The listing builds one solid part. Answer for the finished solid, in the listing's coordinates (mm). Coordinates: 2 decimals unless noted, no trailing zeros. Write each loop counter-clockwise with the first axis right and the second up, starting at its lowest first coordinate (ties: lowest second). Pieces come first, ordered by that corner, then holes.
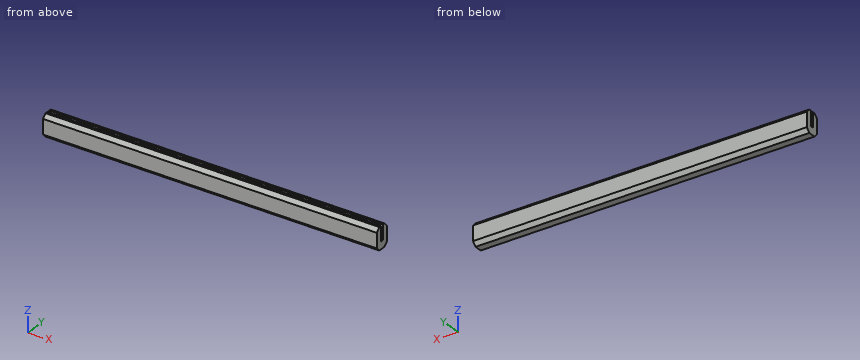
from build123d import *

# Parameters (mm, degrees)
F0_W     = 90
F0_H     = 1.625
F0_H_2   = 0.75
F1_DEPTH = 2
F2_DEPTH = 4
F3_SIZE2 = 1
F3_SIZE  = 1


with BuildPart() as f1:
    # F0 (on Top) → F1 (new body)
    with BuildSketch(Plane.XY):
        with Locations((7.534994, -1.493563)):
            Rectangle(F0_W, F0_H)
        with Locations((7.534994, -0.306063)):
            Rectangle(F0_W, F0_H_2)
        with Locations((7.534994, 0.881437)):
            Rectangle(F0_W, F0_H)
    extrude(amount=-F1_DEPTH)

    # F0 (on Top) → F2 (join)
    with BuildSketch(Plane.XY):
        with Locations((7.534994, 0.881437)):
            Rectangle(F0_W, F0_H)
        with Locations((7.534994, -1.493563)):
            Rectangle(F0_W, F0_H)
    extrude(amount=F2_DEPTH)

    # F3
    f3_edges = [f1.edges().sort_by_distance(p)[0] for p in [
        (7.534994, 1.693937, -2),
        (7.534994, -2.306063, -2),
        (7.534994, 1.693937, 4),
        (7.534994, -2.306063, 4),
    ]]
    chamfer(f3_edges, length=F3_SIZE, length2=F3_SIZE2)


solid = f1.part
1. A flat-ended cylindrical pin translates along its axis: P1, Ø2, axis at x = 1, y = -1.5, coming from the -Z side. Find the tip coordinate at first contact, or state that the pin passes through.
Results found:
P1: stops at z = -2
2. Find the intervals of material crossed by L1, parallel to Y at x = 12, z = 0.05; L2, parallel to Y at x = -10, z = 3.5; L3, parallel to Z at x = 48, y = -0.45, in increasing order.
Results found:
L1: y = -2.31 to -0.68, 0.07 to 1.69
L2: y = -1.81 to -0.68, 0.07 to 1.19
L3: z = -2 to 0
3. Section A-A on x = -22 is taken. Give the vertices of the cut face in (y, z), then the cut area to 3 significant figures.
Results found:
outline: (-2.31, -1) - (-1.31, -2) - (0.69, -2) - (1.69, -1) - (1.69, 3) - (0.69, 4) - (0.07, 4) - (0.07, 0) - (-0.68, 0) - (-0.68, 4) - (-1.31, 4) - (-2.31, 3) - close
area: 19.0 mm2
